Autodesk Inventor part; units mm, degrees
ref_plane "YZ Plane" through (0, 0, 0) normal (1, 0, 0) x (0, 1, 0)
ref_plane "XZ Plane" through (0, 0, 0) normal (0, 1, 0) x (-1, 0, 0)
ref_plane "XY Plane" through (0, 0, 0) normal (0, 0, 1) x (1, 0, 0)
sketch "Sketch1" plane through (0, 0, 0) normal (1, 0, 0) x (0, 1, 0)
  circle A0 centre (0, 0) radius 50.8 construction
  circle A1 centre (82.55, 0) radius 31.75 construction
  circle A2 centre (-82.55, 0) radius 31.75 construction
  circle A3 centre (0, 0) radius 114.3 construction
  circle A4 centre (0, 0) radius 38.1 construction
  arc A5 (38.1, 0) -> (114.3, 0) centre (76.2, 0) ccw construction
  arc A6 (-38.1, 0) -> (139.7, 0) centre (50.8, 0) ccw construction
  line L0 (50.8, -88.9) -> (139.7, -88.9) construction
  line L1 (139.7, -88.9) -> (139.7, 0) construction
  line L2 (139.7, 0) -> (-101.6, 0) construction
  line L3 (-101.6, 0) -> (-101.6, 139.7) construction
  line L4 (-101.6, 139.7) -> (139.7, 139.7) construction
  line L5 (139.7, 139.7) -> (139.7, 0) construction
  arc A7 (11.0716, 139.7) -> (-101.6, 96.52) centre (0, 0) ccw construction
  line L6 (-101.6, 139.7) -> (-101.6, 63.1817) construction
  line L7 (-101.6, 63.1817) -> (-95.25, 63.1817) construction
  arc A8 (-11.0716, 139.7) -> (-101.6, 96.52) centre (0, 0) ccw
  line L8 (-11.0716, 139.7) -> (139.7, 139.7)
  line L9 (139.7, 139.7) -> (139.7, -88.9)
  line L10 (139.7, -88.9) -> (50.8, -88.9)
  arc A9 (-38.1, 0) -> (50.8, -88.9) centre (50.8, 0) ccw
  arc A10 (38.1, 0) -> (-38.1, 0) centre (0, 0) ccw
  arc A11 (38.1, 0) -> (114.3, 0) centre (76.2, 0) ccw
  arc A12 (114.3, 0) -> (-95.25, 63.1817) centre (0, 0) ccw
  line L11 (-95.25, 63.1817) -> (-101.6, 63.1817)
  line L12 (-101.6, 96.52) -> (-101.6, 63.1817)
  dimension "d1" = 63.5
  dimension "d0" = 101.6
  dimension "d2" = 63.5
  dimension "d3" = 82.55
  dimension "d4" = 82.55
  dimension "d5" = 0
  dimension "d6" = 0
  dimension "d7" = 228.6
  dimension "d8" = 76.2
  dimension "d9" = 76.2
  dimension "d10" = 177.8
  dimension "d11" = 88.9
  dimension "d12" = 139.7
  dimension "d13" = 0
  dimension "d14" = 241.3
  dimension "d15" = 139.7
  dimension "d16" = 0
  dimension "d74" = 6.35
  dimension "d75" = 43.18
extrude "Extrusion1" add sketch "Sketch1" along normal blind 3.175
sketch "Sketch2" plane through (3.175, 0, 0) normal (1, 0, 0) x (0, 0, -1)
  arc A0 (0, 38.1) -> (0, -38.1) centre (0, 0) ccw
  arc A1 (0, -38.1) -> (88.9, 50.8) centre (0, 50.8) ccw
  line L0 (88.9, 50.8) -> (88.9, 139.7)
  line L1 (88.9, 139.7) -> (-139.7, 139.7)
  line L2 (-139.7, 139.7) -> (-139.7, -11.0716)
  arc A2 (-139.7, -11.0716) -> (-96.52, -101.6) centre (0, 0) ccw
  line L3 (-96.52, -101.6) -> (-63.1817, -101.6)
  line L4 (-63.1817, -101.6) -> (-63.1817, -95.25)
  arc A3 (0, 114.3) -> (-63.1817, -95.25) centre (0, 0) ccw
  arc A4 (0, 38.1) -> (0, 114.3) centre (0, 76.2) ccw
  line L5 (-63.1817, -101.6) -> (-139.3817, -101.6)
  line L6 (-139.3817, -101.6) -> (-139.3817, -95.25)
  line L7 (-139.3817, -95.25) -> (-63.1817, -95.25)
  line L8 (-63.1817, -95.25) -> (-63.1817, -101.6)
  arc A5 (0, 114.3) -> (-63.1817, -95.25) centre (0, 0) ccw
  line L9 (-63.1817, -101.6) -> (-71.842, -101.6)
  line L10 (-71.842, -101.6) -> (-71.842, -88.9)
  line L11 (-71.842, -88.9) -> (-63.1817, -88.9)
  line L12 (-63.1817, -88.9) -> (-63.1817, -101.6)
  point P0 (0, 0)
  dimension "d24" = 76.2
  dimension "d25" = 6.35
  dimension "d26" = 12.7
extrude "Extrusion2" cut sketch "Sketch2" against normal blind 3.175 contours L11 L12 A3 | A3 L7 L10 | L4 L3 L10 L7 | L10 L3 A2 L7 | A2 L5 L6 L7
sketch "Sketch3" plane through (3.175, 0, 0) normal (1, 0, 0) x (0, 0, -1)
  line L0 (-102.7916, -95.25) -> (-71.842, -95.25)
  line L1 (-71.842, -95.25) -> (-71.842, -88.9)
  arc A0 (0, 114.3) -> (-71.842, -88.9) centre (0, 0) ccw
  arc A1 (0, 38.1) -> (0, 114.3) centre (0, 76.2) ccw
  arc A2 (0, 38.1) -> (0, -38.1) centre (0, 0) ccw
  arc A3 (0, -38.1) -> (88.9, 50.8) centre (0, 50.8) ccw
  line L2 (88.9, 50.8) -> (88.9, 139.7)
  line L3 (88.9, 139.7) -> (-139.7, 139.7)
  line L4 (-139.7, 139.7) -> (-139.7, -11.0716)
  arc A4 (-139.7, -11.0716) -> (-102.7916, -95.25) centre (0, 0) ccw
  point P0 (0, 0)
  point P1 (-127, 127)
  point P2 (76.2, 127)
  point P3 (-95.25, -82.55)
  point P4 (-127, 0)
  dimension "d29" = 12.7
  dimension "d30" = 12.7
  dimension "d31" = 12.7
  dimension "d32" = 12.7
  dimension "d33" = 12.7
  dimension "d34" = 139.7
  dimension "d35" = 95.25
  dimension "d36" = 82.55
hole "Hole1" at (3.175, 127, 127) at (3.175, 127, -76.2) at (3.175, -82.55, 95.25) at (3.175, 0, 127) direction (-1, 0, 0) diameter 6.35 end through all
sketch "Sketch4" plane through (3.175, 0, 0) normal (1, 0, 0) x (0, 0, -1)
  circle A0 centre (-95.25, -82.55) radius 3.175
  circle A1 centre (-127, 127) radius 3.175
  circle A2 centre (76.2, 127) radius 3.175
  circle A3 centre (-127, 0) radius 3.175
  line L0 (-102.7916, -95.25) -> (-71.842, -95.25)
  line L1 (-71.842, -95.25) -> (-71.842, -88.9)
  arc A4 (0, 114.3) -> (-71.842, -88.9) centre (0, 0) ccw
  arc A5 (0, 38.1) -> (0, 114.3) centre (0, 76.2) ccw
  arc A6 (0, 38.1) -> (0, -38.1) centre (0, 0) ccw
  arc A7 (0, -38.1) -> (88.9, 50.8) centre (0, 50.8) ccw
  line L2 (88.9, 50.8) -> (88.9, 139.7)
  line L3 (88.9, 139.7) -> (-139.7, 139.7)
  line L4 (-139.7, 139.7) -> (-139.7, -11.0716)
  arc A8 (-139.7, -11.0716) -> (-102.7916, -95.25) centre (0, 0) ccw
  circle A9 centre (0, 0) radius 9.525
  circle A10 centre (-25.4, 0) radius 2.3813
  circle A11 centre (25.4, 0) radius 2.3813
  point P0 (0, 0)
  dimension "d44" = 0
  dimension "d45" = 0
  dimension "d46" = 25.4
  dimension "d47" = 25.4
  dimension "d55" = 19.05
  dimension "d56" = 4.7625
  dimension "d57" = 4.7625
extrude "Extrusion3" cut sketch "Sketch4" against normal blind 3.175 contours A9 | A10 | A11
sketch "Sketch5" plane through (3.175, 0, 0) normal (1, 0, 0) x (0, 0, -1)
  circle A0 centre (25.4, 0) radius 2.3813
  circle A1 centre (-25.4, 0) radius 2.3813
  circle A2 centre (0, 0) radius 9.525
  circle A3 centre (-95.25, -82.55) radius 3.175
  circle A4 centre (-127, 127) radius 3.175
  circle A5 centre (76.2, 127) radius 3.175
  circle A6 centre (-127, 0) radius 3.175
  line L0 (-102.7916, -95.25) -> (-71.842, -95.25)
  line L1 (-71.842, -95.25) -> (-71.842, -88.9)
  arc A7 (0, 114.3) -> (-71.842, -88.9) centre (0, 0) ccw
  arc A8 (0, 38.1) -> (0, 114.3) centre (0, 76.2) ccw
  arc A9 (0, 38.1) -> (0, -38.1) centre (0, 0) ccw
  arc A10 (0, -38.1) -> (88.9, 50.8) centre (0, 50.8) ccw
  line L2 (88.9, 50.8) -> (88.9, 139.7)
  line L3 (88.9, 139.7) -> (-139.7, 139.7)
  line L4 (-139.7, 139.7) -> (-139.7, -11.0716)
  arc A11 (-139.7, -11.0716) -> (-102.7916, -95.25) centre (0, 0) ccw
  line L5 (-139.7, -11.0716) -> (-139.7, -95.25) construction
  line L6 (-139.7, -95.25) -> (-102.7916, -95.25) construction
  line L7 (-139.7, -95.25) -> (-127, -95.25) construction
  line L8 (-127, -95.25) -> (-127, -82.55) construction
  line L9 (-127, -82.55) -> (-139.7, -82.55) construction
  line L10 (-139.7, -82.55) -> (-139.7, -95.25) construction
  line L11 (-139.7, -11.0716) -> (-139.7, -82.55)
  line L12 (-139.7, -82.55) -> (-127, -95.25)
  line L13 (-127, -95.25) -> (-102.7916, -95.25)
  point P0 (0, 0)
  dimension "d60" = 12.7
  dimension "d61" = 12.7
extrude "Extrusion4" add sketch "Sketch5" against normal blind 3.175 contours L13 L12 L11 A11
sketch "Sketch6" plane through (3.175, 0, 0) normal (1, 0, 0) x (0, 0, -1)
  circle A0 centre (25.4, 0) radius 2.3813
  circle A1 centre (-25.4, 0) radius 2.3813
  circle A2 centre (0, 0) radius 9.525
  circle A3 centre (-95.25, -82.55) radius 3.175
  circle A4 centre (-127, 127) radius 3.175
  circle A5 centre (76.2, 127) radius 3.175
  circle A6 centre (-127, 0) radius 3.175
  line L0 (-127, -95.25) -> (-71.842, -95.25)
  line L1 (-71.842, -95.25) -> (-71.842, -88.9)
  arc A7 (0, 114.3) -> (-71.842, -88.9) centre (0, 0) ccw
  arc A8 (0, 38.1) -> (0, 114.3) centre (0, 76.2) ccw
  arc A9 (0, 38.1) -> (0, -38.1) centre (0, 0) ccw
  arc A10 (0, -38.1) -> (88.9, 50.8) centre (0, 50.8) ccw
  line L2 (88.9, 50.8) -> (88.9, 139.7)
  line L3 (88.9, 139.7) -> (-139.7, 139.7)
  line L4 (-139.7, 139.7) -> (-139.7, -82.55)
  line L5 (-139.7, -82.55) -> (-127, -95.25)
  point P0 (0, 0)
  point P1 (-123.825, -85.725)
  dimension "d64" = 15.875
  dimension "d65" = 9.525
hole "Hole3" at (3.175, -85.725, 123.825) direction (-1, 0, 0) diameter 9.525 end through all
fillet "Fillet1" radius 3.175 2 edges at (1.5875, -95.25, 71.842) (1.5875, -88.9, 71.842)
properties part number "rail gearbox mounting" material "Aluminum 6061"
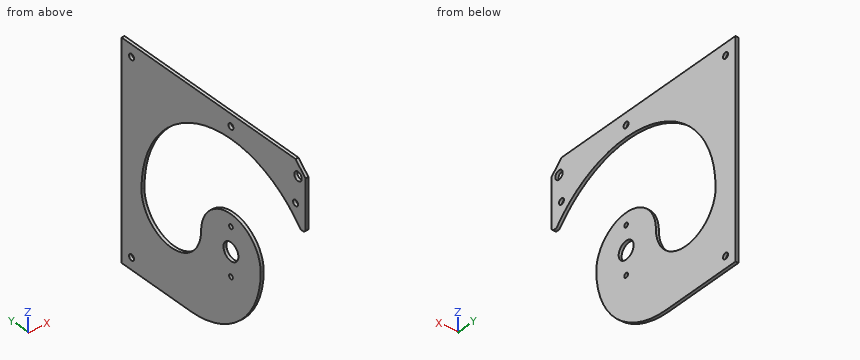
Read the model definition and answer for the solid it produces. Units are mm, in the model's axes. Round coordinates to 2 decimals unless told otherwise and drop trailing zeros. Loops run counter-clockwise (first coordinate to the right, second up) from the corner with the lowest first, then second, coordinate; pieces in that order, holes last.
Q1. Each of these flat-tipped pins is pushed along its axis until it touches: pin 1 (0.8 mm diameter, centred on x = 2, y = -91, fed in from -Z); pin 2 (7.5 mm diameter, centred on y = -85.725, z = 123.825, fed in from -X). Where does it stop, or does it pass through?
Q2. Section A-A on y = 94.5 is taken. Write down the section's boundary in (x, z) (3 decimals).
Q3. Section B-B on x = 1.5 is taken. Give the number of separate pieces and of enclosed holes in the cut face, and give its area (3 significant figures).
Q4. Section D-D on z = 95.25 is taken. Write down the section's boundary in (x, y) (3 decimals), and give its area (3 significant figures).
Q5. Section C-C on z = -33.5 is taken. Write down the section's boundary in (x, y) (3 decimals).
Q6. Consider probe 1 along Y at (x, z) = (0.8, 0) (3 decimals); probe 2 along Y at (x, z) = (1.8, 127) (3 decimals); probe 3 along Z at (x, y) = (1.3, -82.55) (3 decimals). Determine where each line is inside the solid, lowest interval first.
Output:
1. pin 1: stops at z = 71.84
1. pin 2: passes through
2. outline: (0, -88.9) - (3.175, -88.9) - (3.175, -33.417) - (0, -33.417) - close; (0, 64.298) - (3.175, 64.298) - (3.175, 139.7) - (0, 139.7) - close
3. separate pieces: 1
3. enclosed holes: 8
3. area: 26,600 mm2
4. outline: (0, -95.25) - (3.175, -95.25) - (3.175, -85.725) - (0, -85.725) - close; (0, -79.375) - (3.175, -79.375) - (3.175, -63.182) - (0, -63.182) - close; (0, 63.182) - (3.175, 63.182) - (3.175, 139.7) - (0, 139.7) - close
4. area: 325 mm2
5. outline: (0, -31.547) - (3.175, -31.547) - (3.175, 58.052) - (0, 58.052) - close; (0, 94.348) - (3.175, 94.348) - (3.175, 139.7) - (0, 139.7) - close
6. probe 1: y = -38.1 to -9.525, 9.525 to 38.1, 114.3 to 139.7
6. probe 2: y = -95.25 to -89.275, -82.175 to -3.175, 3.175 to 123.825, 130.175 to 139.7
6. probe 3: z = 79.057 to 92.075, 98.425 to 120.275, 127.375 to 139.7
